```python
from build123d import *

# Parameters (mm, degrees)
SKETCH_1_W          = 50
SKETCH_1_H          = 40
SKETCH_1_R          = 1.75
EXTRUDE_1_DEPTH     = 3
FILLET_1_R          = 5
SKETCH_2_W          = 3
SKETCH_2_H          = 40
EXTRUDE_2_DEPTH     = 47
CUT_EXTRUDE_1_REACH = 62.019
SKETCH_3_R          = 1.5
FILLET_2_R          = 5


with BuildPart() as part:
    # 草图1 → 凸台-拉伸1 (new body)
    with BuildSketch(Plane(origin=(0, 0, 0), x_dir=(1, 0, 0), z_dir=(0, 1, 0))):
        Rectangle(SKETCH_1_W, SKETCH_1_H)
        with Locations(Location((-12, 15, 0), (0, 0, 270))):
            Circle(SKETCH_1_R, mode=Mode.SUBTRACT)
        with Locations(Location((12, 15, 0), (0, 0, 270))):
            Circle(SKETCH_1_R, mode=Mode.SUBTRACT)
        with Locations(Location((12, -15, 0), (0, 0, 270))):
            Circle(SKETCH_1_R, mode=Mode.SUBTRACT)
        with Locations(Location((-12, -15, 0), (0, 0, 270))):
            Circle(SKETCH_1_R, mode=Mode.SUBTRACT)
    extrude(amount=EXTRUDE_1_DEPTH)

    # 圆角1
    fillet_1_edges = [part.edges().sort_by_distance(p)[0] for p in [
        (25, 1.5, 20),
        (-25, 1.5, 20),
        (-25, 1.5, -20),
        (25, 1.5, -20),
    ]]
    fillet(fillet_1_edges, radius=FILLET_1_R)

    # 草图2 → 凸台-拉伸2 (add)
    with BuildSketch(Plane(origin=(0, 3, 0), x_dir=(1, 0, 0), z_dir=(0, 1, 0))):
        Rectangle(SKETCH_2_W, SKETCH_2_H)
    extrude(amount=EXTRUDE_2_DEPTH)

    # 草图3 → 切除-拉伸1 (cut, up to next)
    with BuildSketch(Plane.ZY.offset(1.5), mode=Mode.PRIVATE) as cut_extrude_1_sk1:
        with Locations((-10, 46)):
            Circle(SKETCH_3_R)
    cut_extrude_1_tool1 = extrude(cut_extrude_1_sk1.sketch, amount=-CUT_EXTRUDE_1_REACH, mode=Mode.PRIVATE) & part.part
    # 草图3 → 切除-拉伸1 (cut, up to next)
    with BuildSketch(Plane.ZY.offset(1.5), mode=Mode.PRIVATE) as cut_extrude_1_sk2:
        with Locations((10, 46)):
            Circle(SKETCH_3_R)
    cut_extrude_1_tool2 = extrude(cut_extrude_1_sk2.sketch, amount=-CUT_EXTRUDE_1_REACH, mode=Mode.PRIVATE) & part.part
    # 草图3 → 切除-拉伸1 (cut, up to next)
    with BuildSketch(Plane.ZY.offset(1.5), mode=Mode.PRIVATE) as cut_extrude_1_sk3:
        with Locations((10, 26)):
            Circle(SKETCH_3_R)
    cut_extrude_1_tool3 = extrude(cut_extrude_1_sk3.sketch, amount=-CUT_EXTRUDE_1_REACH, mode=Mode.PRIVATE) & part.part
    # 草图3 → 切除-拉伸1 (cut, up to next)
    with BuildSketch(Plane.ZY.offset(1.5), mode=Mode.PRIVATE) as cut_extrude_1_sk4:
        with Locations((-10, 26)):
            Circle(SKETCH_3_R)
    cut_extrude_1_tool4 = extrude(cut_extrude_1_sk4.sketch, amount=-CUT_EXTRUDE_1_REACH, mode=Mode.PRIVATE) & part.part
    add(cut_extrude_1_tool1.solids().sort_by_distance((-1.5, 46, -10))[0], mode=Mode.SUBTRACT)
    add(cut_extrude_1_tool2.solids().sort_by_distance((-1.5, 46, 10))[0], mode=Mode.SUBTRACT)
    add(cut_extrude_1_tool3.solids().sort_by_distance((-1.5, 26, 10))[0], mode=Mode.SUBTRACT)
    add(cut_extrude_1_tool4.solids().sort_by_distance((-1.5, 26, -10))[0], mode=Mode.SUBTRACT)

    # 圆角2
    fillet_2_edges = [part.edges().sort_by_distance(p)[0] for p in [
        (0, 50, -20),
        (0, 50, 20),
    ]]
    fillet(fillet_2_edges, radius=FILLET_2_R)


solid = part.part
```
Design review of the part built by this model. Coordinates are the model's own, in mm. A direction names the side the tool comes from. Round coordinates to 2 decimals unless told otherwise and drop trailing zeros. Write each loop counter-clockwise with the first axis right and the second up, starting at its lowest first coordinate (ties: lowest second). Pieces come first, ordered by that corner, then holes. Notation, with made-up numbers: (85, 7) -> (132, 7) arc R21 ccw to (132, 26) -> close; hole circle Ø4 at (-30.5, 80.25). An arc over 180 degrees is marked (long way). Write item = value, one per line. Start each with the question number.
1) Wall thickness on probe 1 along Y at (x, z) = (0, 10); probe 2 along X at (y, z) = (2.3, -15); probe 3 along X at (y, z) = (10, 14.5): over which ranges is each line inside the solid? List them lowest first. Write a range as from..to.
2) Mouldability with a two-part tool opening along Y and no side actions: class faces 3 (the face through (0, 12, -20)), 4 (the face through (0, 50, 0)), 5 (the face through (-0.021, 44.536, -10.325)), 6 (the face through (-0.021, 44.536, 9.675)) as +Y half, -Y half, draft (parallel to the pull), parting line (faces both ways), or undercut.
3) Tool access review of faces 1 (the face through (13, 3, 0)), 2 (the face through (0, 0, 0)): name each direction out of +Z, -Z, +X, -X, +Y, -Y from which nothing blocks a thin tool from reaching the whole face with its end or side.
4) Take a section at A-A, the plane z = 10. State the section outline as (x, y) points.
5) Clearance check with flat-ended pins moving along their axes: pin 1 (8 mm diameter, centred on y = 38, z = 12.5, fed in from -X); pin 2 (3 mm diameter, centred on x = 12, z = -15, fed in from -Y); pin 3 (3.5 mm diameter, centred on y = 46, z = 10, fed in from +X); pin 4 (4 mm diameter, centred on x = 12, z = 15, fed in from +Y). State where each tip first meets the part, or that it passes through.
6) Take a section at B-B, the plane x = -12. State the section outline as (y, z) points, plus the area to 3 significant figures.
7) Take a section at D-D, the plane z = -1.5. State the section outline as (x, y) points, plus the area to 3 significant figures.
8) Take a section at C-C, the plane y = 46. State the section outline as (x, z) points.
Results list:
q1.probe_1 = 0..24.5, 27.5..44.5, 47.5..50
q1.probe_2 = -25..-13.75, -10.25..10.25, 13.75..25
q1.probe_3 = -1.5..1.5
q2.face_3 = draft
q2.face_4 = +Y half
q2.face_5 = undercut
q2.face_6 = undercut
q3.face_1 = +Z, -Z, +X, +Y
q3.face_2 = +Z, -Z, +X, -X, -Y
q4.outline = (-25, 0) -> (25, 0) -> (25, 3) -> (1.5, 3) -> (1.5, 24.5) -> (-1.5, 24.5) -> (-1.5, 3) -> (-25, 3) -> close; (-1.5, 27.5) -> (1.5, 27.5) -> (1.5, 44.5) -> (-1.5, 44.5) -> close; (-1.5, 47.5) -> (1.5, 47.5) -> (1.5, 50) -> (-1.5, 50) -> close
q5.pin_1 = -1.5
q5.pin_2 = through
q5.pin_3 = 1.5
q5.pin_4 = 3
q6.outline = (0, -20) -> (3, -20) -> (3, -16.75) -> (0, -16.75) -> close; (0, -13.25) -> (3, -13.25) -> (3, 13.25) -> (0, 13.25) -> close; (0, 16.75) -> (3, 16.75) -> (3, 20) -> (0, 20) -> close
q6.area = 99.0 mm²
q7.outline = (-25, 0) -> (25, 0) -> (25, 3) -> (1.5, 3) -> (1.5, 50) -> (-1.5, 50) -> (-1.5, 3) -> (-25, 3) -> close
q7.area = 291 mm²
q8.outline = (-1.5, -19.9) -> (1.5, -19.9) -> (1.5, -11.5) -> (-1.5, -11.5) -> close; (-1.5, -8.5) -> (1.5, -8.5) -> (1.5, 8.5) -> (-1.5, 8.5) -> close; (-1.5, 11.5) -> (1.5, 11.5) -> (1.5, 19.9) -> (-1.5, 19.9) -> close
